from build123d import *

# Parameters (mm, degrees)
SKETCH1_W           = 16.5
SKETCH1_H           = 12
GEARBOX_DEPTH       = 11.3
SKETCH2_R           = 2.5
SHAFTBASE_DEPTH     = 0.5
SHAFT_DEPTH         = 3.1
MOTOR_DEPTH         = 13.9
SKETCH5_W           = 2
SKETCH5_H           = 2
SCREWINSETS_DEPTH   = 1
SKETCH6_R           = 1.25
BACKEXTRUSION_DEPTH = 0.6
FILLETS_R           = 0.5


with BuildPart() as part:
    # Sketch1 → gearbox (new body)
    with BuildSketch(Plane(origin=(0, 0, 0), x_dir=(1, 0, 0), z_dir=(0, 1, 0))):
        with Locations((3.05, 0)):
            Rectangle(SKETCH1_W, SKETCH1_H)
    extrude(amount=-GEARBOX_DEPTH)

    # Sketch2 → shaftbase (add)
    with BuildSketch(Plane(origin=(0, 0, 0), x_dir=(1, 0, 0), z_dir=(0, 1, 0))):
        with Locations(Location((0, 0, 0), (0, 0, 270))):
            Circle(SKETCH2_R)
    extrude(amount=SHAFTBASE_DEPTH)

    # Sketch3 → shaft (add)
    with BuildSketch(Plane(origin=(0, 0.5, 0), x_dir=(1, 0, 0), z_dir=(0, 1, 0))):
        with BuildLine():
            Line((-1.2, 0.981070844), (-1.2, -0.981070844))
            ThreePointArc((-1.2, -0.981070844), (0, -1.55), (1.2, -0.981070844))
            Line((1.2, -0.981070844), (1.2, 0.981070844))
            ThreePointArc((1.2, 0.981070844), (0, 1.55), (-1.2, 0.981070844))
        make_face()
    extrude(amount=SHAFT_DEPTH)

    # Sketch4 → motor (add)
    with BuildSketch(Plane(origin=(11.3, 0, 0), x_dir=(0, 0, -1), z_dir=(1, 0, 0))):
        with BuildLine():
            Line((2.332380758, -11.3), (-2.332380758, -11.3))
            ThreePointArc((-2.332380758, -11.3), (0, -4.5), (2.332380758, -11.3))
        make_face()
    extrude(amount=MOTOR_DEPTH)

    # Sketch5 → screwinsets (cut)
    with BuildSketch(Plane(origin=(0, 0, 0), x_dir=(1, 0, 0), z_dir=(0, 1, 0))):
        with Locations((-4.2, 5)):
            Rectangle(SKETCH5_W, SKETCH5_H)
        with Locations((10.3, 5)):
            Rectangle(SKETCH5_W, SKETCH5_H)
        with Locations((10.3, -5)):
            Rectangle(SKETCH5_W, SKETCH5_H)
        with Locations((-4.2, -5)):
            Rectangle(SKETCH5_W, SKETCH5_H)
    extrude(amount=-SCREWINSETS_DEPTH, mode=Mode.SUBTRACT)

    # Sketch6 → backextrusion (add)
    with BuildSketch(Plane.XZ.offset(11.3)):
        with Locations(Location((5, 0, 0), (0, 0, 90))):
            Circle(SKETCH6_R)
    extrude(amount=BACKEXTRUSION_DEPTH)

    # fillets
    fillets_edges = [part.edges().sort_by_distance(p)[0] for p in [
        (-3.2, -0.5, -6),
        (-5.2, -0.5, -4),
        (-5.2, -0.5, 4),
        (-3.2, -0.5, 6),
        (9.3, -0.5, -6),
        (11.3, -0.5, -4),
        (11.3, -0.5, 4),
        (9.3, -0.5, 6),
        (-3.2, -0.5, -4),
        (9.3, -0.5, 4),
        (9.3, -0.5, -4),
        (-3.2, -0.5, 4),
        (-5.2, -6.15, -6),
        (-5.2, -6.15, 6),
        (11.3, -6.15, -6),
        (11.3, -6.15, 6),
    ]]
    fillet(fillets_edges, radius=FILLETS_R)


solid = part.part
Source: CAD feature listing. Evaluate the final solid. Frame: model axes, mm. A direction names the side the tool comes from. Give positions to 0.01 mm unless a question says otherwise; leave off trailing zeros. Write each loop counter-clockwise with the first axis right and the second up, starting at its lowest first coordinate (ties: lowest second). Pieces come first, ordered by that corner, then holes. Notation, with made-up numbers: M 20.5,28.5 L 69.5,28.5 A12 cw 69.5,50.5 Z; hole C 19,74.5 d2. An arc over 180 degrees is marked long. Answer as a JSON object with one key per item and string values.
Q1. Cut plane A-A, the plane z = 5. Return the cut outline in (x, y).
Geometry check:
{"outline": "M -5.2,-11.3 L 11.3,-11.3 L 11.3,-1 L 9.3,-1 L 9.3,0 L -3.2,0 L -3.2,-1 L -5.2,-1 Z"}
Q2. Ray query, line 1 along Y through (x, z) = (-1, -2.75); line 2 along Y through (x, z) = (-0.5, 0); line 3 along X through (y, z) = (-4.5, -0.5). Return the intervals inside material, ascending.
Geometry check:
{"line 1": "y = -11.3 to 0", "line 2": "y = -11.3 to 3.6", "line 3": "x = -5.2 to 11.3"}
Q3. Cut plane B-B, the plane y = -8.3. Return the cut outline in (x, z).
Geometry check:
{"outline": "M -5.2,-5.5 A0.5 ccw -4.7,-6 L 10.8,-6 A0.5 ccw 11.3,-5.5 L 11.3,-3.8 L 25.2,-3.8 L 25.2,3.8 L 11.3,3.8 L 11.3,5.5 A0.5 ccw 10.8,6 L -4.7,6 A0.5 ccw -5.2,5.5 Z"}
Q4. Cut plane D-D, the plane x = 0. Return the cut outline in (y, z).
Geometry check:
{"outline": "M -11.3,-6 L 0,-6 L 0,-2.5 L 0.5,-2.5 L 0.5,-1.55 L 3.6,-1.55 L 3.6,1.55 L 0.5,1.55 L 0.5,2.5 L 0,2.5 L 0,6 L -11.3,6 Z"}
Q5. Cut plane C-C, the plane x = 5. Return the cut outline in (y, z), then the cut area to 3 significant figures.
Geometry check:
{"outline": "M -11.9,-1.25 L -11.3,-1.25 L -11.3,-6 L 0,-6 L 0,6 L -11.3,6 L -11.3,1.25 L -11.9,1.25 Z", "area": "137 mm^2"}
Q6. Access query for faces 1 (the face through (-4.2, -0.5, 4)), 2 (the face through (10.3, -0.5, -4)), 3 (the face through (0.02, 2.03, -1.55)), 4 (the face through (-3.2, -0.5, -5)), 5 (the face through (18.2, -4.5, 0.1)). Directions: +Z, -Z, +X, -X, +Y, -Y. A direction counts if a zero-diameter tool reaches every point of the face in a straight line with its end or side. Return the directions, or none.
Geometry check:
{"face 1": "+Z, -X, +Y", "face 2": "-Z, +X, +Y", "face 3": "-Z, +Y", "face 4": "-Z, -X, +Y", "face 5": "+X"}
Q7. Contact query for flat-ended pins moving along their axis: P1, Ø0.8, axis at x = -4.5, y = -0.5, coming from the -Z side; P2, Ø0.6, axis at y = 2, z = 0, coming from the -X side; P3, Ø5, axis at x = 6, z = -2.5, coming from the +Y side. Output: stop coordinate, or through.
Geometry check:
{"P1": "stops at z = -4", "P2": "stops at x = -1.2", "P3": "stops at y = 0"}
